Check sheet for the modelled part. Datum: model origin and axes. Units: mm. A direction names the side the tool comes from. Round coordinates to 2 decimals unless told otherwise and drop trailing zeros. Order: outer loops, then holes, each group sorted by start corner. A loop starts at its lowest first (then second) coordinate and runs counter-clockwise, first axis right, second up.
```python
from build123d import *

# Parameters (mm, degrees)
SKETCH1_R           = 7.9375
BOSS_EXTRUDE1_DEPTH = 3.175
SKETCH2_W           = 4.318
SKETCH2_H           = 5.6642
CUT_EXTRUDE1_DEPTH  = 1.27
SKETCH3_R           = 0.508
CUT_EXTRUDE2_DEPTH  = 75.215587445


with BuildPart() as part:
    # Sketch1 → Boss-Extrude1 (new body)
    with BuildSketch(Plane(origin=(0, 0, 0), x_dir=(1, 0, 0), z_dir=(0, 1, 0))):
        Polygon((0, 0), (16.51, 0), (16.51, -3.175), (35.56, -3.175), (35.56, 0), (52.07, 0), (52.07, 9.525), (48.895, 9.525), (48.895, 28.575), (52.07, 28.575), (52.07, 38.1), (45.958497653, 39.823960283), (45.096517511, 36.768209109), (34.095813286, 39.871337619), (34.957793427, 42.927088793), (22.734788732, 46.375009359), (21.872808591, 43.319258185), (7.205202957, 47.456762864), (8.067183099, 50.512514038), (0, 52.788141612), (0, 28.575), (3.175, 28.575), (3.175, 9.525), (0, 9.525), align=None)
        with Locations(Location((12.827, 25.512426191, 0), (0, 0, 270))):
            Circle(SKETCH1_R, mode=Mode.SUBTRACT)
        with Locations(Location((39.243, 25.512426191, 0), (0, 0, 270))):
            Circle(SKETCH1_R, mode=Mode.SUBTRACT)
    extrude(amount=BOSS_EXTRUDE1_DEPTH)

    # Sketch2 → Cut-Extrude1 (cut)
    with BuildSketch(Plane(origin=(0, 3.175, 0), x_dir=(1, 0, 0), z_dir=(0, 1, 0))):
        with Locations((26.035, 14.742826191)):
            Rectangle(SKETCH2_W, SKETCH2_H)
    extrude(amount=-CUT_EXTRUDE1_DEPTH, mode=Mode.SUBTRACT)

    # Sketch3 → Cut-Extrude2 (cut, through all)
    with BuildSketch(Plane(origin=(0, 3.175, 0), x_dir=(1, 0, 0), z_dir=(0, 1, 0))):
        with Locations(Location((17.526, 11.910726191, 0), (0, 0, 270))):
            Circle(SKETCH3_R)
        with Locations(Location((34.544, 11.910726191, 0), (0, 0, 270))):
            Circle(SKETCH3_R)
    extrude(amount=-CUT_EXTRUDE2_DEPTH, mode=Mode.SUBTRACT)


solid = part.part
```
Item 1: Sectioned sample at C-C (y = 1.3). Record the cut outline in (x, z) (1 decimal).
Answer:
outline: (0, -52.8) - (8.1, -50.5) - (7.2, -47.5) - (21.9, -43.3) - (22.7, -46.4) - (35, -42.9) - (34.1, -39.9) - (45.1, -36.8) - (46, -39.8) - (52.1, -38.1) - (52.1, -28.6) - (48.9, -28.6) - (48.9, -9.5) - (52.1, -9.5) - (52.1, 0) - (35.6, 0) - (35.6, 3.2) - (16.5, 3.2) - (16.5, 0) - (0, 0) - (0, -9.5) - (3.2, -9.5) - (3.2, -28.6) - (0, -28.6) - close; hole circle Ø15.9 at (12.8, -25.5); hole circle Ø1 at (17.5, -11.9); hole circle Ø15.9 at (39.2, -25.5); hole circle Ø1 at (34.5, -11.9)
Item 2: Go/stop test with flat-tipped pins: P1, Ø1.6, axis at y = 2, z = -22.5, coming from the -X side (3 decimals); P2, Ø1, axis at x = 1, y = 2, coming from the -Z side; P3, Ø1, axis at y = 2, z = -16.5, coming from the +X side (3 decimals). Record where each tip stops, or that it passes through.
Answer:
P1: stops at x = 3.175
P2: stops at z = -52.65
P3: stops at x = 48.895
Item 3: Access from +Z, -Z, +X, -X, +Y, -Y to the whole of each face (thin tool, end or side, straight path). Record for faces 1 (the flat face through (3.175, 2, -19)), 2 (the flat face through (23.876, 3, -15)), 3 (the flat face through (48.895, 2, -19)), 4 (the flat face through (35.56, 2, 2)).
Answer:
face 1: -X, +Y, -Y
face 2: +Y
face 3: +X, +Y, -Y
face 4: +Z, +X, +Y, -Y
Item 4: Scan lines: line 1 along X through (y, z) = (2.6, -14) (3 decimals); line 2 along X through (y, z) = (2.7, -20) (3 decimals); line 3 along X through (y, z) = (2.3, -11.5) (3 decimals). Record each from-to range of solid material in increasing order.
Answer:
line 1: x = 3.175 to 23.876, 28.194 to 48.895
line 2: x = 3.175 to 7.116, 18.538 to 33.532, 44.954 to 48.895
line 3: x = 3.175 to 17.227, 17.825 to 34.245, 34.843 to 48.895
Item 5: Sectioned sample at D-D (z = -39). Record the cut outline in (x, y) (3 decimals).
Answer:
outline: (0, 0) - (37.185, 0) - (37.185, 3.175) - (0, 3.175) - close; (45.726, 0) - (48.879, 0) - (48.879, 3.175) - (45.726, 3.175) - close
Item 6: Sectioned sample at A-A (x = 13.5). Record the cut outline in (y, z) (1 decimal).
Answer:
outline: (0, -45.7) - (3.2, -45.7) - (3.2, -33.4) - (0, -33.4) - close; (0, -17.6) - (3.2, -17.6) - (3.2, 0) - (0, 0) - close
Item 7: Release check for a two-part mould opening along X. For faces 5 (the flat face through (45.534, 1.565, -38.317)), 6 (the flat face through (49.06, 1.57, -38.95)), 7 (the flat face through (26, 3, -17.575)), 8 (the flat face through (2, 2, -9.525)) record: released by +X, released by -X, zero draft, split by the parting line, or undercut.
Answer:
face 5: undercut
face 6: released by +X
face 7: undercut
face 8: zero draft
Item 8: Sectioned sample at B-B (z = -16.5). Record the cut outline in (x, y) (3 decimals).
Answer:
outline: (3.175, 0) - (48.895, 0) - (48.895, 3.175) - (28.194, 3.175) - (28.194, 1.905) - (23.876, 1.905) - (23.876, 3.175) - (3.175, 3.175) - close
